Work out the finished part from the listing and answer in its coordinate system (mm). Face numbers are marked on the shaded views. A direction names the side the tool comes from. Round coordinates to 2 decimals unless told otherwise and drop trailing zeros. Order: outer loops, then holes, each group sorted by start corner. A loop starts at its lowest first (then second) coordinate and runs counter-clockwise, first axis right, second up. Notation, with made-up numbers: (-29.5, 55) - (-3.5, 55) arc R31 ccw to (-3.5, 87) - close; hole circle Ø6 at (64.25, -34). An arc over 180 degrees is marked (long way). Answer in a Markdown table with one row per item.
from build123d import *

# Parameters (mm, degrees)
SKETCH_1_W      = 40.3
SKETCH_1_H      = 19.5
EXTRUDE_1_DEPTH = 37
SKETCH_2_R      = 2.9
EXTRUDE_2_DEPTH = 3
SKETCH_3_R      = 1.5
EXTRUDE_3_DEPTH = 3
SKETCH_4_W      = 54
SKETCH_4_H      = 19.5
EXTRUDE_4_DEPTH = 2.5
MM_1_D          = 4
MM_1_DEPTH      = 7.5
MM_1_TIP        = 1.201721238


with BuildPart() as part:
    # 草图1 → 凸台-拉伸1 (new body)
    with BuildSketch(Plane.XY):
        Rectangle(SKETCH_1_W, SKETCH_1_H)
    extrude(amount=EXTRUDE_1_DEPTH)

    # 草图2 → 凸台-拉伸2 (add)
    with BuildSketch(Plane.XY.offset(37)):
        with Locations((3, 0)):
            Circle(SKETCH_2_R)
    extrude(amount=EXTRUDE_2_DEPTH)

    # 草图3 → 凸台-拉伸3 (add)
    with BuildSketch(Plane.XY.offset(40)):
        with Locations((3, 0)):
            Circle(SKETCH_3_R)
    extrude(amount=EXTRUDE_3_DEPTH)

    # 草图4 → 凸台-拉伸4 (add)
    with BuildSketch(Plane.XY.offset(27)):
        Rectangle(SKETCH_4_W, SKETCH_4_H)
    extrude(amount=-EXTRUDE_4_DEPTH)

    # 大小mm 暗销孔1
    with Locations(Plane.XY.offset(27)):
        with Locations((-24.315, 5), (-24.315, -5), (24.315, -5), (24.315, 5)):
            Hole(MM_1_D / 2, depth=MM_1_DEPTH)
            with Locations((0, 0, -(MM_1_DEPTH + MM_1_TIP / 2))):  # 118° drill point
                Cone(0, MM_1_D / 2, MM_1_TIP, mode=Mode.SUBTRACT)


solid = part.part
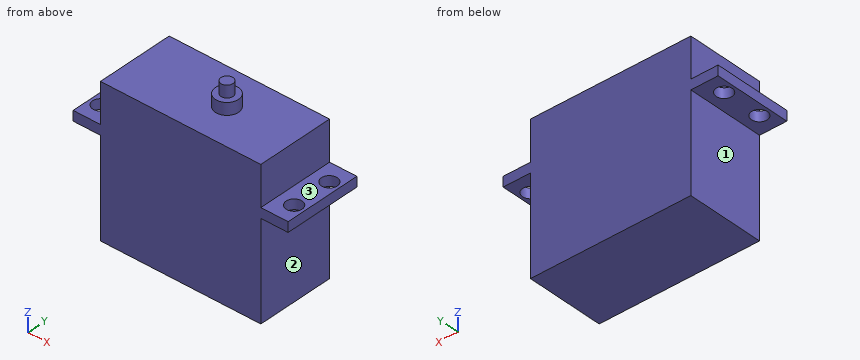
1) Find section C-C, the plane x = 3. Give the vertices of the cut face in (y, z).
Filled in:
| item | result |
|---|---|
| outline | (-9.75, 0) - (9.75, 0) - (9.75, 37) - (2.9, 37) - (2.9, 40) - (1.5, 40) - (1.5, 43) - (-1.5, 43) - (-1.5, 40) - (-2.9, 40) - (-2.9, 37) - (-9.75, 37) - close |
2) Find section B-B, the plane y = 0. Give the vertices of the cut face in (x, z).
Filled in:
| item | result |
|---|---|
| outline | (-27, 24.5) - (-20.15, 24.5) - (-20.15, 0) - (20.15, 0) - (20.15, 24.5) - (27, 24.5) - (27, 27) - (20.15, 27) - (20.15, 37) - (5.9, 37) - (5.9, 40) - (4.5, 40) - (4.5, 43) - (1.5, 43) - (1.5, 40) - (0.1, 40) - (0.1, 37) - (-20.15, 37) - (-20.15, 27) - (-27, 27) - close |
3) Find section D-D, the plane y = 6. Give the vertices of the cut face in (x, z), then the cut area to 3 significant figures.
Filled in:
| item | result |
|---|---|
| outline | (-27, 24.5) - (-26.05, 24.5) - (-26.05, 27) - (-27, 27) - close; (-22.58, 24.5) - (-20.15, 24.5) - (-20.15, 0) - (20.15, 0) - (20.15, 24.5) - (22.58, 24.5) - (22.58, 27) - (20.15, 27) - (20.15, 37) - (-20.15, 37) - (-20.15, 27) - (-22.58, 27) - close; (26.05, 24.5) - (27, 24.5) - (27, 27) - (26.05, 27) - close |
| area | 1,510 mm^2 |
4) Which of the six approach directions +Z, -Z, +X, -X, +Y, -Y give full straight-line access (tool end or side, diameter ignored) to the marked faces 1, 2 and 3?
Filled in:
| item | result |
|---|---|
| face 1 | -Z, -X, +Y, -Y |
| face 2 | -Z, +X, +Y, -Y |
| face 3 | +Z, +X, +Y, -Y |
5) Find the intervals of material crossed by probe 1 along Z at (x, y) = (1, -2.75); probe 2 along X at (y, z) = (-3.75, 7); probe 3 along Z at (x, y) = (4, -1.75), in increasing order. Write a range as from..to.
Filled in:
| item | result |
|---|---|
| probe 1 | z = 0..37 |
| probe 2 | x = -20.15..20.15 |
| probe 3 | z = 0..40 |
6) Each of these flat-tipped pins is pushed along its axis until it touches: pin 1 (5 mm diameter, centred on x = -16.5, y = 7.5, fed in from +Z); pin 2 (6 mm diameter, centred on y = -0.5, z = 6.5, fed in from -X); pin 3 (11 mm diameter, centred on y = 4.5, z = 33.5, fed in from +X). Where does it stop, or does it pass through?
Filled in:
| item | result |
|---|---|
| pin 1 | stops at z = 37 |
| pin 2 | stops at x = -20.15 |
| pin 3 | stops at x = 20.15 |
7) Find section A-A, the plane y = -5. Give the vertices of the cut face in (x, z) (3 decimals).
Filled in:
| item | result |
|---|---|
| outline | (-27, 24.5) - (-26.315, 24.5) - (-26.315, 27) - (-27, 27) - close; (-22.315, 24.5) - (-20.15, 24.5) - (-20.15, 0) - (20.15, 0) - (20.15, 24.5) - (22.315, 24.5) - (22.315, 27) - (20.15, 27) - (20.15, 37) - (-20.15, 37) - (-20.15, 27) - (-22.315, 27) - close; (26.315, 24.5) - (27, 24.5) - (27, 27) - (26.315, 27) - close |
